Can you work these out from the model? Positions are in its coordinate system, mm. A direction names the side the tool comes from. Give positions to 0.01 mm unless a question says otherwise; leave off trailing zeros. Write each loop counter-clockwise with the first axis right and the second up, starting at its lowest first coordinate (ties: lowest second). Pieces come first, ordered by that corner, then holes.
from build123d import *

# Parameters (mm, degrees)
F0_R     = 58
F0_R_2   = 53
F1_DEPTH = 136
F3_DEPTH = 136
F4_W     = 35
F4_H     = 33.777588
F5_DEPTH = 25
F6_W     = 46
F6_H     = 3.5
F7_DEPTH = 136


with BuildPart() as f1:
    # F0 (on Top) → F1 (new body)
    with BuildSketch(Plane.XY):
        Circle(F0_R)
        Circle(F0_R_2, mode=Mode.SUBTRACT)
    extrude(amount=F1_DEPTH)

    # F2 (on Top) → F3 (join)
    with BuildSketch(Plane.XY):
        Polygon((-8.05435, -54.732766), (-30, -45.9545), (-30, -62.025927), (30, -62.025927), (30, -47.670264), (6.974748, -54.732766), align=None)
    extrude(amount=F3_DEPTH)

    # F4 (on face) → F5 (cut)
    with BuildSketch(Plane.XZ.offset(62.025927)):
        with Locations((0, 50)):
            Rectangle(F4_W, F4_H)
        with BuildLine():
            Line((-17.5, 66.888794), (17.5, 66.888794))
            ThreePointArc((17.5, 66.888794), (0, 84.388794), (-17.5, 66.888794))
        make_face()
        with BuildLine():
            ThreePointArc((-17.5, 33.111206), (0, 15.611206), (17.5, 33.111206))
            Line((17.5, 33.111206), (-17.5, 33.111206))
        make_face()
    extrude(amount=-F5_DEPTH, mode=Mode.SUBTRACT)

    # F6 (on face) → F7 (cut)
    with BuildSketch(Plane.XY.offset(136)):
        with Locations((0, -57.525927)):
            Rectangle(F6_W, F6_H)
    extrude(amount=-F7_DEPTH, mode=Mode.SUBTRACT)


solid = f1.part
(1) Imagine slicing it at C-C, the plane x = 0. Write out the boundary of the cut face in (y, z).
Returned:
outline: (-62.03, 0) - (-59.28, 0) - (-59.28, 15.61) - (-62.03, 15.61) - close; (-62.03, 84.39) - (-59.28, 84.39) - (-59.28, 136) - (-62.03, 136) - close; (-55.78, 0) - (-53, 0) - (-53, 15.61) - (-55.78, 15.61) - close; (-55.78, 84.39) - (-53, 84.39) - (-53, 136) - (-55.78, 136) - close; (53, 0) - (58, 0) - (58, 136) - (53, 136) - close
(2) If we mould it in two halves opening along X, with no side actions, what happens to faces 1 (the face through (-17, -51, 0)), 2 (the face through (2.11, 57.96, 67.05)), 3 (the face through (-6.9, 52.55, 67.05))? For each: +X half, -X half, draft (parallel to the pull), parting line (faces both ways), or undercut.
Returned:
face 1: draft
face 2: parting line
face 3: undercut
(3) If I drill on L1, parallel to Y at x = 0, z = 90; L2, parallel to X at y = -56, z = 72.5; L3, parallel to Y at x = 0, z = 75, over which ranges is the centre line in solid material (lowest first)?
Returned:
L1: y = -62.03 to -59.28, -55.78 to -53, 53 to 58
L2: x = -30 to -23, 23 to 30
L3: y = 53 to 58
(4) For faces 4 (the face through (30, -56, 67)), 5 (the face through (0.385, -53.581, 84.385)), 6 (the face through (-30, -56, 67)), 7 (the face through (-5, -59.276, 84)), which set-ups out of +Z, -Z, +X, -X, +Y, -Y let a thin tool reach every point of the face, with its end or its side?
Returned:
face 4: +Z, -Z, +X, -Y
face 5: -Y
face 6: +Z, -Z, -X, -Y
face 7: +Z, -Z
(5) Imagine slicing it at A-A, the plane y = 0. Write out the boundary of the cut face in (x, z).
Returned:
outline: (-58, 0) - (-53, 0) - (-53, 136) - (-58, 136) - close; (53, 0) - (58, 0) - (58, 136) - (53, 136) - close
(6) Imagine slicing it at D-D, the plane x = -26. Write out the boundary of the cut face in (y, z), plus the area to 3 significant figures.
Returned:
outline: (-62.03, 0) - (-46.18, 0) - (-46.18, 136) - (-62.03, 136) - close; (46.18, 0) - (51.85, 0) - (51.85, 136) - (46.18, 136) - close
area: 2,920 mm2
(7) Imagine slicing it at B-B, the plane z = 106. Write out the boundary of the cut face in (x, y).
Returned:
outline: (-30, -62.03) - (30, -62.03) - (30, -49.64) arc R58 ccw (long way) to (-30, -49.64) - close; hole circle Ø106 at (0, 0); hole (-23, -59.28) - (23, -59.28) - (23, -55.78) - (-23, -55.78) - close
(8) Will these pins go through, and if not, where does the flat tip stop? P1, Ø8, axis at y = -40.5, z = 25.5, coming from the -X side; P2, Ø14, axis at x = -1.5, z = 39, coming from the -Y side; P3, Ø2, axis at y = -33.5, z = 38, coming from the +X side.
Returned:
P1: stops at x = -45.07
P2: stops at y = 52.31
P3: stops at x = 48.04
